Read the model definition and answer for the solid it produces. Units are mm, in the model's axes. A direction names the side the tool comes from. Coordinates: 2 decimals unless noted, no trailing zeros. Loops run counter-clockwise (first coordinate to the right, second up) from the corner with the lowest first, then second, coordinate; pieces in that order, holes last. Notation, with made-up numbers: (-0.5, 26) - (5.5, 26) arc R32 cw to (5.5, 53) - close; hole circle Ø2 at (-5.75, 7). An arc over 180 degrees is marked (long way). Use one line per item in the form item = value. Start each with the question number.
1) Which of the six approach directions +Z, -Z, +X, -X, +Y, -Y give full straight-line access (tool end or side, diameter ignored) to faces 4 (the face through (69, 1.7, 42)), 5 (the face through (69, 204.5, 41))?
2) This flat-tipped pin is pushed along its axis until it touches: P1, Ø2, axis at x = 33.5, y = 39, coming from the +Z side. Where does it stop, or does it pass through?
3) The mould has two halves that part along X. Classify faces 1 (the face through (3.2, 201.37, 41.41)), 2 (the face through (71, 1, 2)), 3 (the face through (138.9, 1.43, 40.55)): released by +X, released by -X, zero draft, split by the parting line, or undercut.
4) A cutting plane is placed at C-C (y = 168). Give the vertices of the cut face in (x, z).
5) Consider line 1 (Y direction, x = 58, z = 11); line 2 (X direction, y = 67, z = 19.5); line 3 (Z direction, x = 114, y = 93.5). Determine where each line is inside the solid, lowest interval first.
6) A cutting plane is placed at A-A (x = 68). Give the vertices of the cut face in (y, z).
7) A cutting plane is placed at B-B (z = 45). Give the vertices of the cut face in (x, y), and give its area (3 significant figures).
from build123d import *

# Parameters (mm, degrees)
F0_W         = 140.4
F0_H         = 204.5
F1_DEPTH     = 77.1
F2_W         = 137
F2_H         = 201.1
F3_DEPTH     = 75.4
F4_R         = 5
F5_T1_DEPTH  = 70.4
F5_S5_W      = 5
F5_S5_H      = 5
F5_T6_DEPTH  = 5
F5_S11_W     = 5
F5_S11_H     = 5
F5_T12_DEPTH = 5
F5_S17_W     = 5
F5_S17_H     = 5
F5_T18_DEPTH = 5
F5_S23_W     = 5
F5_S23_H     = 5
F5_T24_DEPTH = 5
F5_T27_DEPTH = 84.6
F5_S31_W     = 5
F5_S31_H     = 5
F5_T32_DEPTH = 5
F5_S37_W     = 5
F5_S37_H     = 5
F5_T38_DEPTH = 5
F5_S43_W     = 5
F5_S43_H     = 5
F5_T44_DEPTH = 5
F5_S49_W     = 5
F5_S49_H     = 5
F5_T50_DEPTH = 5


# Not quite as in the source:
# - a fillet or chamfer that OpenCascade refuses, or shapes differently, is made with other operations: its cross-section is extruded or revolved along the edge and cut away or added


with BuildPart() as f1:
    # F0 (on Top) → F1 (new body)
    with BuildSketch(Plane.XY):
        with Locations((70.2, 102.25)):
            Rectangle(F0_W, F0_H)
    extrude(amount=F1_DEPTH)

    # F2 (on face) → F3 (cut)
    with BuildSketch(Plane.XY.offset(77.1)):
        with Locations((70.2, 102.25)):
            Rectangle(F2_W, F2_H)
    extrude(amount=-F3_DEPTH, mode=Mode.SUBTRACT)

    # F4
    f4_edges = [f1.edges().sort_by_distance(p)[0] for p in [
        (70.2, 202.8, 1.7),
        (1.7, 102.25, 1.7),
        (70.2, 1.7, 1.7),
        (138.7, 102.25, 1.7),
        (0, 102.25, 0),
        (70.2, 0, 0),
        (140.4, 102.25, 0),
        (70.2, 204.5, 0),
    ]]
    fillet(f4_edges, radius=F4_R)

    # F5: fillet of radius 5 on 8 edges, made by hand

    # F5_s2 → F5_t1 (join)
    with BuildSketch(Plane.XY.offset(6.7)):
        with BuildLine():
            ThreePointArc((133.7, 202.8), (137.2355339059, 201.3355339059), (138.7, 197.8))
            Line((138.7, 197.8), (138.7, 202.8))
            Line((138.7, 202.8), (133.7, 202.8))
        make_face()
        with BuildLine():
            ThreePointArc((6.7, 202.8), (3.1644660941, 201.3355339059), (1.7, 197.8))
            Line((1.7, 197.8), (1.7, 202.8))
            Line((1.7, 202.8), (6.7, 202.8))
        make_face()
        with BuildLine():
            ThreePointArc((1.7, 6.7), (3.1644660941, 3.1644660941), (6.7, 1.7))
            Line((6.7, 1.7), (1.7, 1.7))
            Line((1.7, 1.7), (1.7, 6.7))
        make_face()
        with BuildLine():
            ThreePointArc((133.7, 1.7), (137.2355339059, 3.1644660941), (138.7, 6.7))
            Line((138.7, 6.7), (138.7, 1.7))
            Line((138.7, 1.7), (133.7, 1.7))
        make_face()
    extrude(amount=F5_T1_DEPTH)


with BuildPart() as f5_tool4:
    # F5_s5 → F5_t6 (new body)
    with BuildSketch(Plane.XZ.offset(-6.7)):
        with Locations((136.2, 4.2)):
            Rectangle(F5_S5_W, F5_S5_H)
    extrude(amount=F5_T6_DEPTH)

    # F5_s7 → F5_t8 (revolve, cut)
    with BuildSketch(Plane(origin=(133.7, 6.7, 6.7), x_dir=(-0.7071067812, 0, 0.7071067812), z_dir=(0.7071067812, 0, 0.7071067812))):
        with BuildLine():
            ThreePointArc((0, -5), (5, 0), (0, 5))
            Line((0, 5), (0, -5))
        make_face()
    revolve(axis=Axis((133.7, 6.7, 6.7), (0, -1, 0)), mode=Mode.SUBTRACT)


with BuildPart() as f1_1:
    add(f1.part)

    # F5_t3: union F5_tool4
    add(f5_tool4.part)


with BuildPart() as f5_tool10:
    # F5_s11 → F5_t12 (new body)
    with BuildSketch(Plane.YZ.offset(6.7)):
        with Locations((4.2, 4.2)):
            Rectangle(F5_S11_W, F5_S11_H)
    extrude(amount=-F5_T12_DEPTH)

    # F5_s13 → F5_t14 (revolve, cut)
    with BuildSketch(Plane(origin=(6.7, 6.7, 6.7), x_dir=(0, 0.7071067812, 0.7071067812), z_dir=(0, -0.7071067812, 0.7071067812))):
        with BuildLine():
            ThreePointArc((0, -5), (5, 0), (0, 5))
            Line((0, 5), (0, -5))
        make_face()
    revolve(axis=Axis((6.7, 6.7, 6.7), (-1, 0, 0)), mode=Mode.SUBTRACT)


with BuildPart() as f1_2:
    add(f1_1.part)

    # F5_t9: union F5_tool10
    add(f5_tool10.part)


with BuildPart() as f5_tool16:
    # F5_s17 → F5_t18 (new body)
    with BuildSketch(Plane.XZ.offset(-197.8)):
        with Locations((4.2, 4.2)):
            Rectangle(F5_S17_W, F5_S17_H)
    extrude(amount=-F5_T18_DEPTH)

    # F5_s19 → F5_t20 (revolve, cut)
    with BuildSketch(Plane(origin=(6.7, 197.8, 6.7), x_dir=(0.7071067812, 0, 0.7071067812), z_dir=(-0.7071067812, 0, 0.7071067812))):
        with BuildLine():
            ThreePointArc((0, -5), (5, 0), (0, 5))
            Line((0, 5), (0, -5))
        make_face()
    revolve(axis=Axis((6.7, 197.8, 6.7), (0, 1, 0)), mode=Mode.SUBTRACT)


with BuildPart() as f1_3:
    add(f1_2.part)

    # F5_t15: union F5_tool16
    add(f5_tool16.part)


with BuildPart() as f5_tool22:
    # F5_s23 → F5_t24 (new body)
    with BuildSketch(Plane.XZ.offset(-197.8)):
        with Locations((136.2, 4.2)):
            Rectangle(F5_S23_W, F5_S23_H)
    extrude(amount=-F5_T24_DEPTH)

    # F5_s25 → F5_t26 (revolve, cut)
    with BuildSketch(Plane(origin=(133.7, 197.8, 6.7), x_dir=(-0.7071067812, 0, 0.7071067812), z_dir=(-0.7071067812, 0, -0.7071067812))):
        with BuildLine():
            ThreePointArc((0, -5), (5, 0), (0, 5))
            Line((0, 5), (0, -5))
        make_face()
    revolve(axis=Axis((133.7, 197.8, 6.7), (0, 1, 0)), mode=Mode.SUBTRACT)


with BuildPart() as f1_4:
    add(f1_3.part)

    # F5_t21: union F5_tool22
    add(f5_tool22.part)

    # F5_s28 → F5_t27 (cut)
    with BuildSketch(Plane.XY.offset(5)):
        with BuildLine():
            ThreePointArc((0, 5), (1.4644660941, 1.4644660941), (5, 0))
            Line((5, 0), (0, 0))
            Line((0, 0), (0, 5))
        make_face()
        with BuildLine():
            ThreePointArc((135.4, 0), (138.9355339059, 1.4644660941), (140.4, 5))
            Line((140.4, 5), (140.4, 0))
            Line((140.4, 0), (135.4, 0))
        make_face()
        with BuildLine():
            ThreePointArc((135.4, 204.5), (138.9355339059, 203.0355339059), (140.4, 199.5))
            Line((140.4, 199.5), (140.4, 204.5))
            Line((140.4, 204.5), (135.4, 204.5))
        make_face()
        with BuildLine():
            ThreePointArc((0, 199.5), (1.4644660941, 203.0355339059), (5, 204.5))
            Line((5, 204.5), (0, 204.5))
            Line((0, 204.5), (0, 199.5))
        make_face()
    extrude(amount=F5_T27_DEPTH, mode=Mode.SUBTRACT)


with BuildPart() as f5_tool30:
    # F5_s31 → F5_t32 (new body)
    with BuildSketch(Plane.YZ.offset(5)):
        with Locations((202, 2.5)):
            Rectangle(F5_S31_W, F5_S31_H)
    extrude(amount=-F5_T32_DEPTH)

    # F5_s33 → F5_t34 (revolve, cut)
    with BuildSketch(Plane(origin=(5, 199.5, 5), x_dir=(0, -0.7071067812, 0.7071067812), z_dir=(0, -0.7071067812, -0.7071067812))):
        with BuildLine():
            ThreePointArc((0, -5), (5, 0), (0, 5))
            Line((0, 5), (0, -5))
        make_face()
    revolve(axis=Axis((5, 199.5, 5), (-1, 0, 0)), mode=Mode.SUBTRACT)


with BuildPart() as f1_5:
    add(f1_4.part)

    # F5_t29: cut F5_tool30
    add(f5_tool30.part, mode=Mode.SUBTRACT)


with BuildPart() as f5_tool36:
    # F5_s37 → F5_t38 (new body)
    with BuildSketch(Plane.XZ.offset(-199.5)):
        with Locations((137.9, 2.5)):
            Rectangle(F5_S37_W, F5_S37_H)
    extrude(amount=-F5_T38_DEPTH)

    # F5_s39 → F5_t40 (revolve, cut)
    with BuildSketch(Plane(origin=(135.4, 199.5, 5), x_dir=(-0.7071067812, 0, 0.7071067812), z_dir=(-0.7071067812, 0, -0.7071067812))):
        with BuildLine():
            ThreePointArc((0, -5), (5, 0), (0, 5))
            Line((0, 5), (0, -5))
        make_face()
    revolve(axis=Axis((135.4, 199.5, 5), (0, 1, 0)), mode=Mode.SUBTRACT)


with BuildPart() as f1_6:
    add(f1_5.part)

    # F5_t35: cut F5_tool36
    add(f5_tool36.part, mode=Mode.SUBTRACT)


with BuildPart() as f5_tool42:
    # F5_s43 → F5_t44 (new body)
    with BuildSketch(Plane.XZ.offset(-5)):
        with Locations((137.9, 2.5)):
            Rectangle(F5_S43_W, F5_S43_H)
    extrude(amount=F5_T44_DEPTH)

    # F5_s45 → F5_t46 (revolve, cut)
    with BuildSketch(Plane(origin=(135.4, 5, 5), x_dir=(-0.7071067812, 0, 0.7071067812), z_dir=(0.7071067812, 0, 0.7071067812))):
        with BuildLine():
            ThreePointArc((0, -5), (5, 0), (0, 5))
            Line((0, 5), (0, -5))
        make_face()
    revolve(axis=Axis((135.4, 5, 5), (0, -1, 0)), mode=Mode.SUBTRACT)


with BuildPart() as f1_7:
    add(f1_6.part)

    # F5_t41: cut F5_tool42
    add(f5_tool42.part, mode=Mode.SUBTRACT)


with BuildPart() as f5_tool48:
    # F5_s49 → F5_t50 (new body)
    with BuildSketch(Plane.YZ.offset(5)):
        with Locations((2.5, 2.5)):
            Rectangle(F5_S49_W, F5_S49_H)
    extrude(amount=-F5_T50_DEPTH)

    # F5_s51 → F5_t52 (revolve, cut)
    with BuildSketch(Plane(origin=(5, 5, 5), x_dir=(0, 0.7071067812, 0.7071067812), z_dir=(0, -0.7071067812, 0.7071067812))):
        with BuildLine():
            ThreePointArc((0, -5), (5, 0), (0, 5))
            Line((0, 5), (0, -5))
        make_face()
    revolve(axis=Axis((5, 5, 5), (-1, 0, 0)), mode=Mode.SUBTRACT)


with BuildPart() as f1_8:
    add(f1_7.part)

    # F5_t47: cut F5_tool48
    add(f5_tool48.part, mode=Mode.SUBTRACT)


solid = f1_8.part
Found:
q1.face_4 = +Z
q1.face_5 = +Z, -Z, +X, -X, +Y
q2.P1 = 1.7
q3.face_1 = undercut
q3.face_2 = zero draft
q3.face_3 = released by +X
q4.outline = (0, 5) arc R5 ccw to (5, 0) - (135.4, 0) arc R5 ccw to (140.4, 5) - (140.4, 77.1) - (138.7, 77.1) - (138.7, 6.7) arc R5 cw to (133.7, 1.7) - (6.7, 1.7) arc R5 cw to (1.7, 6.7) - (1.7, 77.1) - (0, 77.1) - close
q5.line_1 = 0 to 1.7, 202.8 to 204.5
q5.line_2 = 0 to 1.7, 138.7 to 140.4
q5.line_3 = 0 to 1.7
q6.outline = (0, 5) arc R5 ccw to (5, 0) - (199.5, 0) arc R5 ccw to (204.5, 5) - (204.5, 77.1) - (202.8, 77.1) - (202.8, 6.7) arc R5 cw to (197.8, 1.7) - (6.7, 1.7) arc R5 cw to (1.7, 6.7) - (1.7, 77.1) - (0, 77.1) - close
q7.outline = (0, 5) arc R5 ccw to (5, 0) - (135.4, 0) arc R5 ccw to (140.4, 5) - (140.4, 199.5) arc R5 ccw to (135.4, 204.5) - (5, 204.5) arc R5 ccw to (0, 199.5) - close; hole (1.7, 6.7) arc R5 ccw to (6.7, 1.7) - (133.7, 1.7) arc R5 ccw to (138.7, 6.7) - (138.7, 197.8) arc R5 ccw to (133.7, 202.8) - (6.7, 202.8) arc R5 ccw to (1.7, 197.8) - close
q7.area = 1,160 mm^2
